```python
from build123d import *

# Parameters (mm, degrees)
SKETCH_1_R          = 10.5
SKETCH_1_R_2        = 6
EXTRUDE_1_DEPTH     = 4
SKETCH_2_R          = 11.5
SKETCH_2_R_2        = 6
EXTRUDE_2_DEPTH     = 1
SKETCH_3_R          = 9.5
SKETCH_3_R_2        = 9
CUT_EXTRUDE_1_DEPTH = 0.2
CUT_EXTRUDE_START   = -0.2
SKETCH_4_R          = 9.5
SKETCH_4_R_2        = 9
CUT_EXTRUDE_2_DEPTH = 0.2


with BuildPart() as part:
    # 草图1 → 凸台-拉伸1 (new body)
    with BuildSketch(Plane(origin=(0, 0, 0), x_dir=(1, 0, 0), z_dir=(0, 1, 0))):
        with Locations(Location((0, 0, 0), (0, 0, 270))):
            Circle(SKETCH_1_R)
        with Locations(Location((0, 0, 0), (0, 0, 270))):
            Circle(SKETCH_1_R_2, mode=Mode.SUBTRACT)
    extrude(amount=EXTRUDE_1_DEPTH)

    # 草图2 → 凸台-拉伸2 (add)
    with BuildSketch(Plane(origin=(0, 4, 0), x_dir=(1, 0, 0), z_dir=(0, 1, 0))):
        with Locations(Location((0, 0, 0), (0, 0, 270))):
            Circle(SKETCH_2_R)
        with Locations(Location((0, 0, 0), (0, 0, 270))):
            Circle(SKETCH_2_R_2, mode=Mode.SUBTRACT)
    extrude(amount=EXTRUDE_2_DEPTH)

    # 草图3 → 切除-拉伸1 (cut)
    with BuildSketch(Plane.XZ):
        with Locations(Location((0, 0, 0), (0, 0, 270))):
            Circle(SKETCH_3_R)
        with Locations(Location((0, 0, 0), (0, 0, 270))):
            Circle(SKETCH_3_R_2, mode=Mode.SUBTRACT)
    extrude(amount=-CUT_EXTRUDE_1_DEPTH, mode=Mode.SUBTRACT)

    # 草图4 → 切除-拉伸2 (cut)
    with BuildSketch(Plane(origin=(0, 5, 0), x_dir=(1, 0, 0), z_dir=(0, 1, 0)).offset(CUT_EXTRUDE_START)):
        with Locations(Location((0, 0, 0), (0, 0, 90))):
            Circle(SKETCH_4_R)
        with Locations(Location((0, 0, 0), (0, 0, 90))):
            Circle(SKETCH_4_R_2, mode=Mode.SUBTRACT)
    extrude(amount=CUT_EXTRUDE_2_DEPTH, mode=Mode.SUBTRACT)


solid = part.part
```
Read the model definition and answer for the solid it produces. Units are mm, in the model's axes. A direction names the side the tool comes from. Give positions to 0.01 mm unless a question says otherwise; leave off trailing zeros. Write each loop counter-clockwise with the first axis right and the second up, starting at its lowest first coordinate (ties: lowest second). Pieces come first, ordered by that corner, then holes. Notation, with made-up numbers: (80, -39.5) -> (107, -39.5) arc R27 ccw to (107, -20.5) -> close; hole circle Ø3 at (-32, 44.25). An arc over 180 degrees is marked (long way). Answer as a JSON object with one key per item and string values.
1) Straight lines are drawn through the part: probe 1 along X at (y, z) = (4.95, 0); probe 2 along X at (y, z) = (0.1, 0); probe 3 along X at (y, z) = (3.4, 0). For each, find the intervals that lie inside material, in ascending order. Write a range as from..to.
Findings below:
{"probe 1": "x = -11.5..-9.5, -9..-6, 6..9, 9.5..11.5", "probe 2": "x = -10.5..-9.5, -9..-6, 6..9, 9.5..10.5", "probe 3": "x = -10.5..-6, 6..10.5"}
2) Flat-ended cylindrical pins translate along their axes: pin 1 Ø3 at (y, z) = (3.5, 3.5) entering from -X; pin 2 Ø1.5 at (y, z) = (4, 7.5) entering from +X; pin 3 Ø3 at (x, y) = (-1, 1) entering from +Z; pin 4 Ø9.5 at (x, z) = (0, 0) entering from +Y. Find the tip coordinate at first contact, or state that the pin passes through.
Findings below:
{"pin 1": "stops at x = -11.31", "pin 2": "stops at x = 9.31", "pin 3": "stops at z = 10.5", "pin 4": "passes through"}
3) Section C-C on z = -7 is taken. Write down the section's boundary in (x, y).
Findings below:
{"outline": "(-9.12, 4) -> (-7.83, 4) -> (-7.83, 0) -> (-6.42, 0) -> (-6.42, 0.2) -> (-5.66, 0.2) -> (-5.66, 0) -> (5.66, 0) -> (5.66, 0.2) -> (6.42, 0.2) -> (6.42, 0) -> (7.83, 0) -> (7.83, 4) -> (9.12, 4) -> (9.12, 5) -> (6.42, 5) -> (6.42, 4.8) -> (5.66, 4.8) -> (5.66, 5) -> (-5.66, 5) -> (-5.66, 4.8) -> (-6.42, 4.8) -> (-6.42, 5) -> (-9.12, 5) -> close"}
4) Section D-D on y = 1.55 is taken. Write down the section's boundary in (x, z), then the cut area to 3 significant figures.
Findings below:
{"outline": "circle Ø21 at (0, 0); hole circle Ø12 at (0, 0)", "area": "233 mm^2"}
5) Section B-B on z = 0 is taken. Write down the section's boundary in (x, y), then the cut area to 3 significant figures.
Findings below:
{"outline": "(-11.5, 4) -> (-10.5, 4) -> (-10.5, 0) -> (-9.5, 0) -> (-9.5, 0.2) -> (-9, 0.2) -> (-9, 0) -> (-6, 0) -> (-6, 5) -> (-9, 5) -> (-9, 4.8) -> (-9.5, 4.8) -> (-9.5, 5) -> (-11.5, 5) -> close; (6, 0) -> (9, 0) -> (9, 0.2) -> (9.5, 0.2) -> (9.5, 0) -> (10.5, 0) -> (10.5, 4) -> (11.5, 4) -> (11.5, 5) -> (9.5, 5) -> (9.5, 4.8) -> (9, 4.8) -> (9, 5) -> (6, 5) -> close", "area": "46.6 mm^2"}
6) A tool of negligible diameter and unlimited length cuts with its end or side. For faces 1 (the flat face through (-10.2, 4, 3.4)), 2 (the cylindrical face through (9.7, 4.49, 6.18)), 3 (the flat face through (7, 4.8, 6)), from which of +Z, -Z, +X, -X, +Y, -Y can it reach the whole face along a straight path? Write none if from no direction.
Findings below:
{"face 1": "-Y", "face 2": "+Y, -Y", "face 3": "+Y"}
7) Section A-A on x = 0 is taken. Write down the section's boundary in (y, z), then the cut area to 3 significant figures.
Findings below:
{"outline": "(0, -10.5) -> (4, -10.5) -> (4, -11.5) -> (5, -11.5) -> (5, -9.5) -> (4.8, -9.5) -> (4.8, -9) -> (5, -9) -> (5, -6) -> (0, -6) -> (0, -9) -> (0.2, -9) -> (0.2, -9.5) -> (0, -9.5) -> close; (0, 6) -> (5, 6) -> (5, 9) -> (4.8, 9) -> (4.8, 9.5) -> (5, 9.5) -> (5, 11.5) -> (4, 11.5) -> (4, 10.5) -> (0, 10.5) -> (0, 9.5) -> (0.2, 9.5) -> (0.2, 9) -> (0, 9) -> close", "area": "46.6 mm^2"}
8) For a pull along Z with two mould halves and no side action, classify faces 4 (the flat face through (-7, 0.2, 6)), 5 (the cylindrical face through (3.2, 2, 10)), 6 (the flat face through (-6, 0, 2)) as pulls with the +Z half, pulls with the -Z half, needs draft (parallel to the pull), parting line crosses it, or undercut.
Findings below:
{"face 4": "undercut", "face 5": "parting line crosses it", "face 6": "needs draft"}
